```python
from build123d import *

# Parameters (mm, degrees)
SKETCH_1_W                       = 550
SKETCH_1_H                       = 800
SM_BASE_FLANGE_1_DEPTH           = 2
SKETCH_6_W                       = 40
SKETCH_6_H                       = 130
CUT_EXTRUDE_1_DEPTH              = 10
FILLET_1_R                       = 5
SKETCH_7_W                       = 1
SKETCH_7_H                       = 845.505579408
CUT_EXTRUDE_2_DEPTH              = 10
SKETCH_8_W                       = 313.779033263
SKETCH_8_H                       = 811.185879887
CUT_EXTRUDE_3_DEPTH              = 10
SM_EDGE_FLANGE_1_STRIP_W         = 9.4732
SM_EDGE_FLANGE_1_STRIP_H         = 2
SM_EDGE_FLANGE_1_STRIP_CUT_DEPTH = 800
SM_EDGE_FLANGE_1_DEPTH           = 800
FILLET_2_R                       = 5
HOLE_WIZARD_7_0_7_1_D            = 7
CUT_EXTRUDE_4_DEPTH              = 10
HOLE_WIZARD_6_0_6_1_D            = 6
PATTERN_LINEAR_1_COUNT           = 6
PATTERN_LINEAR_1_PITCH           = 150


# Sheet-metal steps are written as plain solids
with BuildPart() as part:
    # Sketch 1 → 基体-法兰1 (new body)
    with BuildSketch(Plane.XY):
        Rectangle(SKETCH_1_W, SKETCH_1_H)
    extrude(amount=-SM_BASE_FLANGE_1_DEPTH)

    # 草图6 → 切除-拉伸1 (cut)
    with BuildSketch(Plane.XY):
        with Locations((255, 335)):
            Rectangle(SKETCH_6_W, SKETCH_6_H)
        with Locations((255, -335)):
            Rectangle(SKETCH_6_W, SKETCH_6_H)
    extrude(amount=-CUT_EXTRUDE_1_DEPTH, mode=Mode.SUBTRACT)

    # 圆角1
    fillet_1_edges = [part.edges().sort_by_distance(p)[0] for p in [
        (275, 270, -1),
        (235, 270, -1),
        (235, 400, -1),
        (275, -270, -1),
        (235, -400, -1),
        (235, -270, -1),
        (-275, 400, -1),
        (-275, -400, -1),
    ]]
    fillet(fillet_1_edges, radius=FILLET_1_R)

    # 草图7 → 切除-拉伸2 (cut)
    with BuildSketch(Plane.XY):
        Rectangle(SKETCH_7_W, SKETCH_7_H)
    extrude(amount=-CUT_EXTRUDE_2_DEPTH, mode=Mode.SUBTRACT)


with BuildPart() as cut_extrude_2_piece_1:
    # of the separate pieces the step leaves, piece 1, a body of its own (cut_extrude_2_pieces)
    add(part.part.solids().sort_by_distance((-0.5, -400, 0))[0])

    # 边线-法兰1 strip (across the edge) → 边线-法兰1 strip cut (cut)
    with BuildSketch(Plane(origin=(-0.5, -400, 0), x_dir=(-1, 0, 0), z_dir=(0, 1, 0))):
        with Locations((-2, -1)):
            Rectangle(SM_EDGE_FLANGE_1_STRIP_W, SM_EDGE_FLANGE_1_STRIP_H)
    extrude(amount=SM_EDGE_FLANGE_1_STRIP_CUT_DEPTH, mode=Mode.SUBTRACT)

    # 边线-法兰1 section (across the edge) → 边线-法兰1 (add)
    with BuildSketch(Plane(origin=(-0.5, -400, 0), x_dir=(-1, 0, 0), z_dir=(0, 1, 0))):
        with BuildLine():
            Line((0, 0.7366), (0, 23))
            Line((0, 23), (2, 23))
            Line((2, 23), (2, 0.7366))
            ThreePointArc((2, 0.7366), (2.215745145, 0.215745145), (2.7366, 0))
            Line((2.7366, 0), (2.7366, -2))
            ThreePointArc((2.7366, -2), (0.801531583, -1.198468417), (0, 0.7366))
        make_face()
    extrude(amount=SM_EDGE_FLANGE_1_DEPTH)

    # 圆角2
    fillet_2_edges = [cut_extrude_2_piece_1.edges().sort_by_distance(p)[0] for p in [
        (-1.5, -400, 23),
        (-1.5, 400, 23),
    ]]
    fillet(fillet_2_edges, radius=FILLET_2_R)

    # Ø7.0 (7) 直径孔1 (through all)
    with Locations(Plane.XY):
        with Locations((-235, 380), (-135, 380), (-35, 380), (-35, -380), (-135, -380), (-235, -380)):
            Hole(HOLE_WIZARD_7_0_7_1_D / 2)

    # 草图15 → 切除-拉伸4 (cut)
    with BuildSketch(Plane.XY):
        with BuildLine():
            Line((-238.5, 375), (-238.5, 385))
            ThreePointArc((-238.5, 385), (-235, 388.5), (-231.5, 385))
            Line((-231.5, 385), (-231.5, 375))
            ThreePointArc((-231.5, 375), (-235, 371.5), (-238.5, 375))
        make_face()
        with BuildLine():
            Line((-138.5, 375), (-138.5, 385))
            ThreePointArc((-138.5, 385), (-135, 388.5), (-131.5, 385))
            Line((-131.5, 385), (-131.5, 375))
            ThreePointArc((-131.5, 375), (-135, 371.5), (-138.5, 375))
        make_face()
        with BuildLine():
            Line((-38.5, 375), (-38.5, 385))
            ThreePointArc((-38.5, 385), (-35, 388.5), (-31.5, 385))
            Line((-31.5, 385), (-31.5, 375))
            ThreePointArc((-31.5, 375), (-35, 371.5), (-38.5, 375))
        make_face()
        with BuildLine():
            Line((-238.5, -385), (-238.5, -375))
            ThreePointArc((-238.5, -375), (-235, -371.5), (-231.5, -375))
            Line((-231.5, -375), (-231.5, -385))
            ThreePointArc((-231.5, -385), (-235, -388.5), (-238.5, -385))
        make_face()
        with BuildLine():
            Line((-138.5, -385), (-138.5, -375))
            ThreePointArc((-138.5, -375), (-135, -371.5), (-131.5, -375))
            Line((-131.5, -375), (-131.5, -385))
            ThreePointArc((-131.5, -385), (-135, -388.5), (-138.5, -385))
        make_face()
        with BuildLine():
            Line((-38.5, -385), (-38.5, -375))
            ThreePointArc((-38.5, -375), (-35, -371.5), (-31.5, -375))
            Line((-31.5, -375), (-31.5, -385))
            ThreePointArc((-31.5, -385), (-35, -388.5), (-38.5, -385))
        make_face()
    extrude(amount=-CUT_EXTRUDE_4_DEPTH, mode=Mode.SUBTRACT)

    # Ø6.0 (6) 直径孔1 (through all)
    with Locations(Plane.ZY.offset(2.5)):
        with Locations((13, 375)):
            hole_wizard_6_0_6_1 = Hole(HOLE_WIZARD_6_0_6_1_D / 2)

    # 阵列(线性)1: Ø6.0 (6) 直径孔1 ×6
    with Locations(*[(0, -i * PATTERN_LINEAR_1_PITCH, 0) for i in range(1, PATTERN_LINEAR_1_COUNT)]):
        add(hole_wizard_6_0_6_1, mode=Mode.SUBTRACT)


with BuildPart() as cut_extrude_2_piece_2:
    # of the separate pieces the step leaves, piece 2, a body of its own (cut_extrude_2_pieces)
    add(part.part.solids().sort_by_distance((230, -400, 0))[0])

    # 草图8 → 切除-拉伸3 (cut)
    with BuildSketch(Plane.XY):
        with Locations((157.389516632, -5.592939943)):
            Rectangle(SKETCH_8_W, SKETCH_8_H)
    extrude(amount=-CUT_EXTRUDE_3_DEPTH, mode=Mode.SUBTRACT)


solid = cut_extrude_2_piece_1.part
```
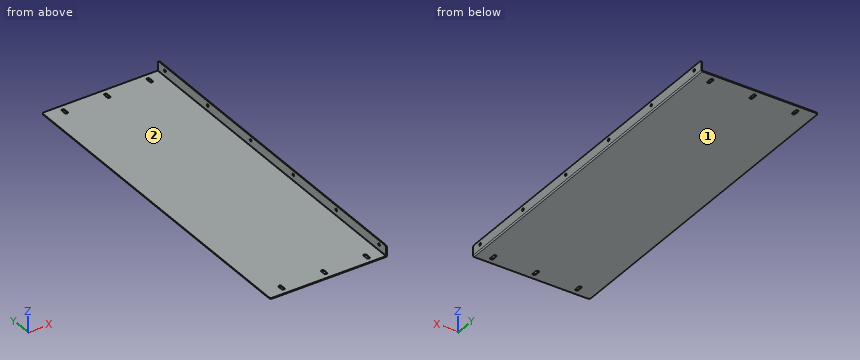
Design review of the part built by this model. Coordinates are the model's own, in mm. Face numbers are marked on the shaded views. A direction names the side the tool comes from. Round coordinates to 2 decimals unless told otherwise and drop trailing zeros. Write each loop counter-clockwise with the first axis right and the second up, starting at its lowest first coordinate (ties: lowest second). Pieces come first, ordered by that corner, then holes.
Item 1: We need section A-A on y = 253. Write out the cut boundary in (x, z), and give its area (3 significant figures).
Item 2: Clearance check with flat-ended pins moving along their axes: pin 1 Ø1 at (y, z) = (-382.5, -1) entering from +X; pin 2 Ø6 at (x, y) = (-29, 66.5) entering from +Z; pin 3 Ø1 at (y, z) = (382, -1.5) entering from +X. State where each tip first meets the part, or that it passes through.
Item 3: We need section B-B on x = -197. Write out the cut boundary in (y, z).
Item 4: For probe 1 along X at (y, z) = (95.5, 10.5); probe 2 along Z at (x, y) = (-53.5, 215.5); probe 3 along Z at (x, y) = (-1.45, 375), list the stretches that pass through material, from the lowest coordinate up.
Item 5: For the marked faces 1 and 2, list the 3-axis set-ups (+Z, -Z, +X, -X, +Y, -Y) from which the entire face can be reached by the end or side of a thin tool; tool diameter is ignored.
Returned:
1. outline: (-275, -2) - (-3.24, -2) arc R2.74 ccw to (-0.5, 0.74) - (-0.5, 23) - (-2.5, 23) - (-2.5, 0.74) arc R0.74 cw to (-3.24, 0) - (-275, 0) - close
1. area: 594 mm2
2. pin 1: stops at x = -0.8
2. pin 2: stops at z = 0
2. pin 3: stops at x = -1.12
3. outline: (-400, -2) - (400, -2) - (400, 0) - (-400, 0) - close
4. probe 1: x = -2.5 to -0.5
4. probe 2: z = -2 to 0
4. probe 3: z = -1.34 to 10, 16 to 23
5. face 1: -Z, +X, -X, +Y, -Y
5. face 2: +Z, -X, +Y, -Y
